Geometry check sheet. Reference: the model listing, model coordinates, mm. Round coordinates to 2 decimals unless told otherwise and drop trailing zeros. Loops run counter-clockwise (first coordinate to the right, second up) from the corner with the lowest first, then second, coordinate; pieces in that order, holes last. Notation, with made-up numbers: (25, 54) -> (32, 54) arc R20 ccw to (32, 64) -> close; hole circle Ø4 at (-13.5, -19). An arc over 180 degrees is marked (long way). Use one line per item in the form item = value.
from build123d import *

# Parameters (mm, degrees)
BASE_R                   = 6.35
BOSS_EXTRU_1_BASE_DEPTH  = 1
PATIN_R                  = 5.85
BOSS_EXTRU_2_PATIN_DEPTH = 2.5
BOSS_EXTRU_2_PATIN_TAPER = 10
CONG_1_0_5MM_PATIN_R     = 0.5


with BuildPart() as part:
    # Base → Boss.-Extru.1_Base (new body)
    with BuildSketch(Plane.XY):
        Circle(BASE_R)
    extrude(amount=BOSS_EXTRU_1_BASE_DEPTH)

    # Patin → Boss.-Extru.2_Patin (add)
    with BuildSketch(Plane.XY.offset(1)):
        Circle(PATIN_R)
    extrude(amount=BOSS_EXTRU_2_PATIN_DEPTH, taper=BOSS_EXTRU_2_PATIN_TAPER)

    # Congé1_0.5mm_Patin
    cong_1_0_5mm_patin_edges = [part.edges().sort_by_distance(p)[0] for p in [
        (-5.409182548, 0, 3.5),
    ]]
    fillet(cong_1_0_5mm_patin_edges, radius=CONG_1_0_5MM_PATIN_R)


solid = part.part
1. Section check C-C (z = 0.45). Record the boundary of the cut face in (x, y).
Return value:
outline = circle Ø12.7 at (0, 0)
2. Material ranges on line 1 along Y through (x, z) = (1, 0.3); line 2 along X through (y, z) = (2.25, 2.7); line 3 along X through (y, z) = (1, 1.6), recorded low to high.
Return value:
line_1 = -6.27 to 6.27
line_2 = -5.07 to 5.07
line_3 = -5.66 to 5.66
3. Section check D-D (z = 2.65). Record the boundary of the cut face in (x, y), then the cut area to 3 significant figures.
Return value:
outline = circle Ø11.12 at (0, 0)
area = 97.1 mm2
4. Gauge pin test, flat end, axial feed: pin 1 (2 mm diameter, centred on x = 3, z = 1.5, fed in from -Y). Record the tip position at first contact, or that the pin passes through.
Return value:
pin_1 = -5.98
5. Section check A-A (y = 0). Record the boundary of the cut face in (x, z), then the cut area to 3 significant figures.
Return value:
outline = (-6.35, 0) -> (6.35, 0) -> (6.35, 1) -> (5.85, 1) -> (5.48, 3.09) arc R0.5 ccw to (4.99, 3.5) -> (-4.99, 3.5) arc R0.5 ccw to (-5.48, 3.09) -> (-5.85, 1) -> (-6.35, 1) -> close
area = 40.8 mm2
